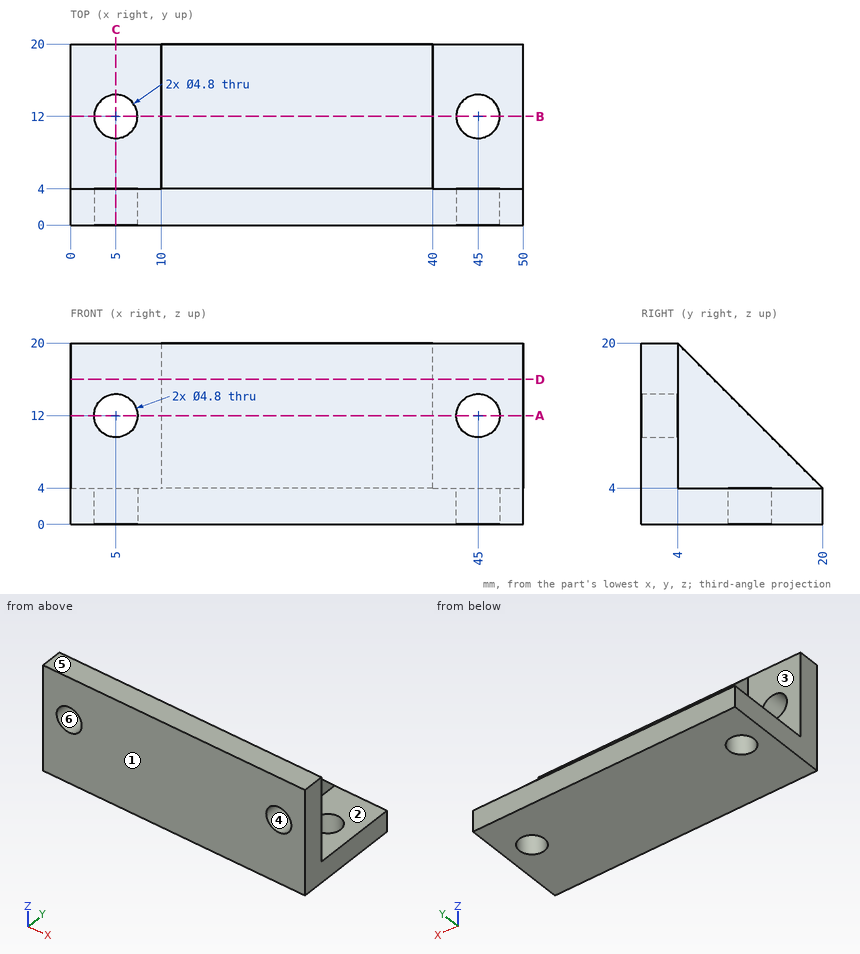
Can you work these out from the drawing? Everything is in mm from the part's minimum corner. A direction names the side the tool comes from. Coordinates: 2 decimals unless noted, no trailing zeros. Write each loop counter-clockwise with the first axis right and the second up, starting at its lowest first coordinate (ties: lowest second). Pieces come first, ordered by that corner, then holes. Notation, with made-up numbers: (18, 19.25) -> (71, 19.25) arc R23 ccw to (71, 32.25) -> close; hole circle Ø11 at (-17, 47.5). An arc over 180 degrees is marked (long way). Return JSON: item names as keys, results as strings.
(1) I'm going to push flat-ended pins straight in: pin 1 (4.5 mm diameter, centred on x = 5, y = 12, fed in from +Z); pin 2 (8 mm diameter, centred on y = 5.5, z = 11.5, fed in from -X); pin 3 (5 mm diameter, centred on x = 16.5, y = 16.5, fed in from +Z); pin 4 (5 mm diameter, centred on x = 43.5, y = 12.5, fed in from +Z). Where does each tip first touch, or does it pass through?
Numbers:
{"pin 1": "passes through", "pin 2": "stops at x = 0", "pin 3": "stops at z = 10", "pin 4": "stops at z = 4"}
(2) We'd pull the mould along Z, two halves only. Please class the marked faces 3, 4, 5 and 6: +Z half, -Z half, draft (parallel to the pull), parting line (faces both ways), or undercut.
Numbers:
{"face 3": "draft", "face 4": "undercut", "face 5": "+Z half", "face 6": "undercut"}
(3) I need wall thicknesses on L1, parallel to Z at x = 45, y = 2.95; L2, parallel to X at y = 13, z = 7.5. Which ranges of each line are inside material? Lowest first, please.
Numbers:
{"L1": "z = 0 to 9.6, 14.4 to 20", "L2": "x = 10 to 40"}
(4) Imagine slicing it at C-C, the plane x = 5. Please give me the cut outline in (y, z).
Numbers:
{"outline": "(0, 0) -> (9.6, 0) -> (9.6, 4) -> (4, 4) -> (4, 9.6) -> (0, 9.6) -> close; (0, 14.4) -> (4, 14.4) -> (4, 20) -> (0, 20) -> close; (14.4, 0) -> (20, 0) -> (20, 4) -> (14.4, 4) -> close"}
(5) Imagine slicing it at A-A, the plane z = 12. Please give me the cut outline in (x, y).
Numbers:
{"outline": "(0, 0) -> (2.6, 0) -> (2.6, 4) -> (0, 4) -> close; (7.4, 0) -> (42.6, 0) -> (42.6, 4) -> (40, 4) -> (40, 12) -> (10, 12) -> (10, 4) -> (7.4, 4) -> close; (47.4, 0) -> (50, 0) -> (50, 4) -> (47.4, 4) -> close"}
(6) Which directions (+Z, -Z, +X, -X, +Y, -Y) give clear straight access to the entire face, cutting with the end or side of a thin tool? Please do the marked faces 1 and 2.
Numbers:
{"face 1": "+Z, -Z, +X, -X, -Y", "face 2": "+Z, +X, +Y"}
(7) Imagine slicing it at D-D, the plane z = 16. Please give me the cut outline in (x, y), then the cut area to 3 significant figures.
Numbers:
{"outline": "(0, 0) -> (50, 0) -> (50, 4) -> (40, 4) -> (40, 8) -> (10, 8) -> (10, 4) -> (0, 4) -> close", "area": "320 mm2"}
